Model file for the job. Use its own axes, mm. Round coordinates to 2 decimals unless told otherwise and drop trailing zeros. Order: outer loops, then holes, each group sorted by start corner. A loop starts at its lowest first (then second) coordinate and runs counter-clockwise, first axis right, second up. Notation, with made-up numbers: (60.25, 3) - (109.25, 3) arc R18 cw to (109.25, 16) - close; hole circle Ø3 at (48, 13). An arc over 180 degrees is marked (long way). Use one line per item in the form item = value.
from build123d import *
from OCP.BRepFilletAPI import BRepFilletAPI_MakeChamfer

# Parameters (mm, degrees)
SKETCH1_R           = 3.125
BOSS_EXTRUDE1_DEPTH = 5
CHAMFER1_SIZE       = 2.5
CHAMFER1_SIZE2      = 5
CHAMFER2_SIZE       = 3.75
CHAMFER2_SIZE2      = 12.5


with BuildPart() as part:
    # Sketch1 → Boss-Extrude1 (new body)
    with BuildSketch(Plane(origin=(0, 0, 0), x_dir=(1, 0, 0), z_dir=(0, 1, 0))):
        with BuildLine():
            Line((0, -12.5), (0, 12.5))
            Line((0, 12.5), (-47.5, 12.5))
            ThreePointArc((-47.5, 12.5), (-60, 0), (-47.5, -12.5))
            Line((-47.5, -12.5), (0, -12.5))
        make_face()
        with Locations(Location((-47.5, 0, 0), (0, 0, 270))):
            Circle(SKETCH1_R, mode=Mode.SUBTRACT)
        with Locations(Location((-37.5, 0, 0), (0, 0, 270))):
            Circle(SKETCH1_R, mode=Mode.SUBTRACT)
        with Locations(Location((-27.5, 0, 0), (0, 0, 270))):
            Circle(SKETCH1_R, mode=Mode.SUBTRACT)
        with Locations(Location((-17.5, 0, 0), (0, 0, 270))):
            Circle(SKETCH1_R, mode=Mode.SUBTRACT)
    extrude(amount=BOSS_EXTRUDE1_DEPTH)

    # Chamfer1: one chamfer whose edges measure the first distance from different faces: ONE call of the kernel's chamfer builder (chamfer() names one face for all edges)
    chamfer1_edges_1 = [part.edges().sort_by_distance(p)[0] for p in [
        (-23.75, 5, -12.5),
    ]]
    chamfer1_side_1 = [part.faces().sort_by_distance(p)[0] for p in [
        (-23.75, 2.5, -12.5),
    ]]
    chamfer1_edges_2 = [part.edges().sort_by_distance(p)[0] for p in [
        (-60, 5, 0),
    ]]
    chamfer1_side_2 = [part.faces().sort_by_distance(p)[0] for p in [
        (-60, 2.5, 0),
    ]]
    chamfer1_edges_3 = [part.edges().sort_by_distance(p)[0] for p in [
        (-23.75, 5, 12.5),
    ]]
    chamfer1_side_3 = [part.faces().sort_by_distance(p)[0] for p in [
        (-23.75, 2.5, 12.5),
    ]]
    chamfer1 = BRepFilletAPI_MakeChamfer(part.part.solid().wrapped)
    for e in chamfer1_edges_1:
        chamfer1.Add(CHAMFER1_SIZE, CHAMFER1_SIZE2, e.wrapped, chamfer1_side_1[0].wrapped)  # the first distance lies on this face
    for e in chamfer1_edges_2:
        chamfer1.Add(CHAMFER1_SIZE, CHAMFER1_SIZE2, e.wrapped, chamfer1_side_2[0].wrapped)  # the first distance lies on this face
    for e in chamfer1_edges_3:
        chamfer1.Add(CHAMFER1_SIZE, CHAMFER1_SIZE2, e.wrapped, chamfer1_side_3[0].wrapped)  # the first distance lies on this face
    add(Compound.cast(chamfer1.Shape()), mode=Mode.REPLACE)

    # Chamfer2
    chamfer2_edges = [part.edges().sort_by_distance(p)[0] for p in [
        (0, 5, 0),
    ]]
    chamfer2_side = [part.faces().sort_by_distance(p)[0] for p in [
        (0, 2.314814815, 0),
    ]]
    chamfer(chamfer2_edges, length=CHAMFER2_SIZE, length2=CHAMFER2_SIZE2, reference=chamfer2_side[0])


solid = part.part
(1) Slice it at B-B on x = -27.5. Give the cut face in (y, z) (3 decimals).
Report:
outline = (0, -12.5) - (2.5, -12.5) - (5, -7.5) - (5, -3.125) - (0, -3.125) - close; (0, 3.125) - (5, 3.125) - (5, 7.5) - (2.5, 12.5) - (0, 12.5) - close
(2) Slice it at D-D on x = -6. Give the cut face in (y, z), then the cut area to 3 significant figures.
Report:
outline = (0, -12.5) - (2.5, -12.5) - (3.05, -11.4) - (3.05, 11.4) - (2.5, 12.5) - (0, 12.5) - close
area = 75.6 mm2
(3) Slice it at A-A on z = 0. Give the cut face in (x, y) (3 decimals), then the cut area to 3 significant figures.
Report:
outline = (-60, 0) - (-50.625, 0) - (-50.625, 5) - (-55, 5) - (-60, 2.5) - close; (-44.375, 0) - (-40.625, 0) - (-40.625, 5) - (-44.375, 5) - close; (-34.375, 0) - (-30.625, 0) - (-30.625, 5) - (-34.375, 5) - close; (-24.375, 0) - (-20.625, 0) - (-20.625, 5) - (-24.375, 5) - close; (-14.375, 0) - (0, 0) - (0, 1.25) - (-12.5, 5) - (-14.375, 5) - close
area = 145 mm2
(4) Probe probe 1 along X at (y, z) = (1.15, 0) (3 decimals); probe 2 along Z at (x, y) = (-28, 0.9); probe 3 along Z at (x, y) = (-29, 0.65). List the from-to ranges inside material, lowest first. Write a range as [from, to].
Report:
probe_1 = [-60, -50.625], [-44.375, -40.625], [-34.375, -30.625], [-24.375, -20.625], [-14.375, 0]
probe_2 = [-12.5, -3.08], [3.08, 12.5]
probe_3 = [-12.5, -2.74], [2.74, 12.5]
(5) Pull direction Z, two halves, no side cores. Call faces 1 (the face through (-44.4, 2.5, -0.4)), 2 (the face through (-30, 0, -3)), 3 (the face through (-55.2, 4.9, -0.2)): released by +Z, released by -Z, zero draft, split by the parting line, or undercut.
Report:
face_1 = undercut
face_2 = zero draft
face_3 = split by the parting line
(6) Pin check, flat tips, straight feed: pin 1 (2 mm diameter, centred on x = -20, z = 10, fed in from -Y); pin 2 (1.5 mm diameter, centred on x = -53, y = 3.5, fed in from +Z); pin 3 (5 mm diameter, centred on x = -37.5, z = 0, fed in from -Y); pin 4 (1 mm diameter, centred on x = -21, z = -8.5, fed in from +Y). Stop position of each tip, or through.
Report:
pin_1 = 0
pin_2 = 10.71
pin_3 = through
pin_4 = 4.75
(7) Slice it at C-C on y = 4.2. Give the cut face in (x, z) (3 decimals).
Report:
outline = (-47.5, -9.1) - (-9.833, -9.1) - (-9.833, 9.1) - (-47.5, 9.1) arc R9.1 ccw to start; hole circle Ø6.25 at (-47.5, 0); hole circle Ø6.25 at (-37.5, 0); hole circle Ø6.25 at (-27.5, 0); hole circle Ø6.25 at (-17.5, 0)
